from build123d import *

# Parameters (mm, degrees)
SKETCH1_W               = 8
SKETCH1_H               = 8
BOSS_EXTRUDE1_DEPTH     = 3
CUT_EXTRUDE1_DEPTH      = 12.704699911
CUT_EXTRUDE1_DEPTH_BACK = 12.704699911
CUT_EXTRUDE2_DEPTH      = 11
SKETCH4_R               = 1.75
CUT_EXTRUDE3_DEPTH      = 0.4
SKETCH5_W               = 8
SKETCH5_H               = 1
BOSS_EXTRUDE2_DEPTH     = 2
FILLET1_R               = 4
SKETCH6_W               = 1.153846154
SKETCH6_H               = 1.153846154
CUT_EXTRUDE4_DEPTH      = 0.4


with BuildPart() as part:
    # Sketch1 → Boss-Extrude1 (new body)
    with BuildSketch(Plane(origin=(0, 0, 0), x_dir=(1, 0, 0), z_dir=(0, 1, 0))):
        with Locations((4, 4)):
            Rectangle(SKETCH1_W, SKETCH1_H)
    extrude(amount=BOSS_EXTRUDE1_DEPTH)

    # Sketch2 → Cut-Extrude1 (cut, two sides: drawn at the far end of the back side and taken through both)
    with BuildSketch(Plane.XY.offset(-CUT_EXTRUDE1_DEPTH_BACK)):
        Polygon((0, 0), (0.6, 3), (0, 3), align=None)
        Polygon((8, 0), (7.4, 3), (8, 3), align=None)
    extrude(amount=CUT_EXTRUDE1_DEPTH + CUT_EXTRUDE1_DEPTH_BACK, mode=Mode.SUBTRACT)

    # Sketch3 → Cut-Extrude2 (cut)
    with BuildSketch(Plane(origin=(0, 0, 0), x_dir=(0, 0, -1), z_dir=(1, 0, 0))):
        Polygon((0, 0), (0.6, 3), (0, 3), align=None)
        Polygon((8, 3), (7.4, 3), (8, 0), align=None)
    extrude(amount=CUT_EXTRUDE2_DEPTH, mode=Mode.SUBTRACT)

    # Sketch4 → Cut-Extrude3 (cut)
    with BuildSketch(Plane.XZ):
        with Locations(Location((4, -3.75, 0), (0, 0, 270))):
            Circle(SKETCH4_R)
    extrude(amount=-CUT_EXTRUDE3_DEPTH, mode=Mode.SUBTRACT)

    # Sketch5 → Boss-Extrude2 (add)
    with BuildSketch(Plane.XZ):
        with Locations((4, -7.5)):
            Rectangle(SKETCH5_W, SKETCH5_H)
    extrude(amount=BOSS_EXTRUDE2_DEPTH)

    # Fillet1
    # the kernel refuses this fillet: 4 mm, written as the material it takes off along each edge
    with BuildSketch(Plane(origin=(8, -2, -16.660254038), x_dir=(0, 1, 0), z_dir=(0, 0, 1)), Plane(origin=(0, -2, 1.660254038), x_dir=(0, 1, 0), z_dir=(0, 0, -1))) as fillet1_piece_1:
        with BuildLine():
            CenterArc((4, 3.464101615), FILLET1_R, 180, 60)
            Line((0, 3.464101615), (-0.08, 3.464101615))
            Line((-0.08, 3.464101615), (-0.08, 0))
            Line((-0.08, 0), (0, -0.08))
            ThreePointArc((0, -0.08), (1, -0.08), (1.96, -0.069282032))
            Line((1.96, -0.069282032), (2, 0))
        make_face()
    extrude(amount=18.320508076, mode=Mode.SUBTRACT)

    # Sketch6 → Cut-Extrude4 (cut)
    with BuildSketch(Plane(origin=(0, 3, 0), x_dir=(1, 0, 0), z_dir=(0, 1, 0))):
        with Locations((4.058809338, 4.067977948)):
            Rectangle(SKETCH6_W, SKETCH6_H)
    extrude(amount=-CUT_EXTRUDE4_DEPTH, mode=Mode.SUBTRACT)


solid = part.part
Here's how the part is built. I have some questions about the finished solid (model axes, mm). A direction names the side the tool comes from. Round coordinates to 2 decimals unless told otherwise and drop trailing zeros. Order: outer loops, then holes, each group sorted by start corner. A loop starts at its lowest first (then second) coordinate and runs counter-clockwise, first axis right, second up. Notation, with made-up numbers: M 0,19.25 L 58,19.25 A26 cw 58,43.25 Z; hole C 47,57 d2. An arc over 180 degrees is marked long. Return JSON: item names as keys, results as strings. Group by question number.
1. If we section it at B-B on x = 7: List the corners of the cut face in (y, z) for me.
2. On a 3-axis mill with a long thin cutter (end or side, diameter ignored), from which of +Z, -Z, +X, -X, +Y, -Y can I reach the whole of each face in a straight line? I mean faces 4 (the face through (4, 0.4, -4)), 5 (the face through (0.3, 1.5, -4.1)), 6 (the face through (4, 2.6, -4)), 7 (the face through (3.9, 1.5, -0.3)), 8 (the face through (4, -1, -7)). Say none if no direction works.
3. If we section it at A-A on z = -3.75: List the corners of the cut face in (x, y) for me.
4. If we section it at C-C on y = 2.05: List the corners of the cut face in (x, z) for me, then the cut area to 3 significant figures.
5. I'm going to push flat-ended pins straight in: pin 1 Ø3 at (x, z) = (4.5, -3) entering from -Y; pin 2 Ø1.5 at (x, y) = (2.5, 2) entering from +Z; pin 3 Ø1 at (x, y) = (6, -1) entering from +Z. Where does each tip first touch, or does it pass through?
6. If we section it at D-D on x = 4: List the corners of the cut face in (y, z) for me.
7. If we mould it in two halves opening along Z, with no side actions, what happens to faces 1 (the face through (4, -1, -8)), 2 (the face through (2.94, 0.2, -2.36)), 3 (the face through (6.51, -1.48, -7.51))? For each: pulls with the +Z half, pulls with the -Z half, needs draft (parallel to the pull), parting line crosses it, or undercut.
8. Please list where these lines run through material, in increasing order: probe 1 along Y at (x, z) = (2, -3); probe 2 along Z at (x, y) = (6.25, -0.1); probe 3 along X at (y, z) = (0.15, -3.75).
Reply:
{
 "1": {"outline": "M -1.15,-8 L 0,-8 L 3,-7.4 L 3,-0.6 L 0,0 L 0,-7 L -1.15,-7 Z"},
 "2": {"face 4": "-Y", "face 5": "+Z, -Z, -X, +Y", "face 6": "+Y", "face 7": "+Z, +X, -X, +Y", "face 8": "+Z, +X, -X, -Y"},
 "3": {"outline": "M 0,0 L 2.25,0 L 2.25,0.4 L 5.75,0.4 L 5.75,0 L 8,0 L 7.4,3 L 4.64,3 L 4.64,2.6 L 3.48,2.6 L 3.48,3 L 0.6,3 Z"},
 "4": {"outline": "M 0.41,-7.59 L 7.59,-7.59 L 7.59,-0.41 L 0.41,-0.41 Z", "area": "51.6 mm^2"},
 "5": {"pin 1": "y = 0", "pin 2": "z = -0.25", "pin 3": "z = -7"},
 "6": {"outline": "M -2,-8 L 0,-8 L 3,-7.4 L 3,-4.64 L 2.6,-4.64 L 2.6,-3.49 L 3,-3.49 L 3,-0.6 L 0,0 L 0,-2 L 0.4,-2 L 0.4,-5.5 L 0,-5.5 L 0,-7 L -2,-7 Z"},
 "7": {"face 1": "pulls with the -Z half", "face 2": "undercut", "face 3": "needs draft"},
 "8": {"probe 1": "0 to 3", "probe 2": "-8 to -7", "probe 3": "0.03 to 2.25, 5.75 to 7.97"}
}
